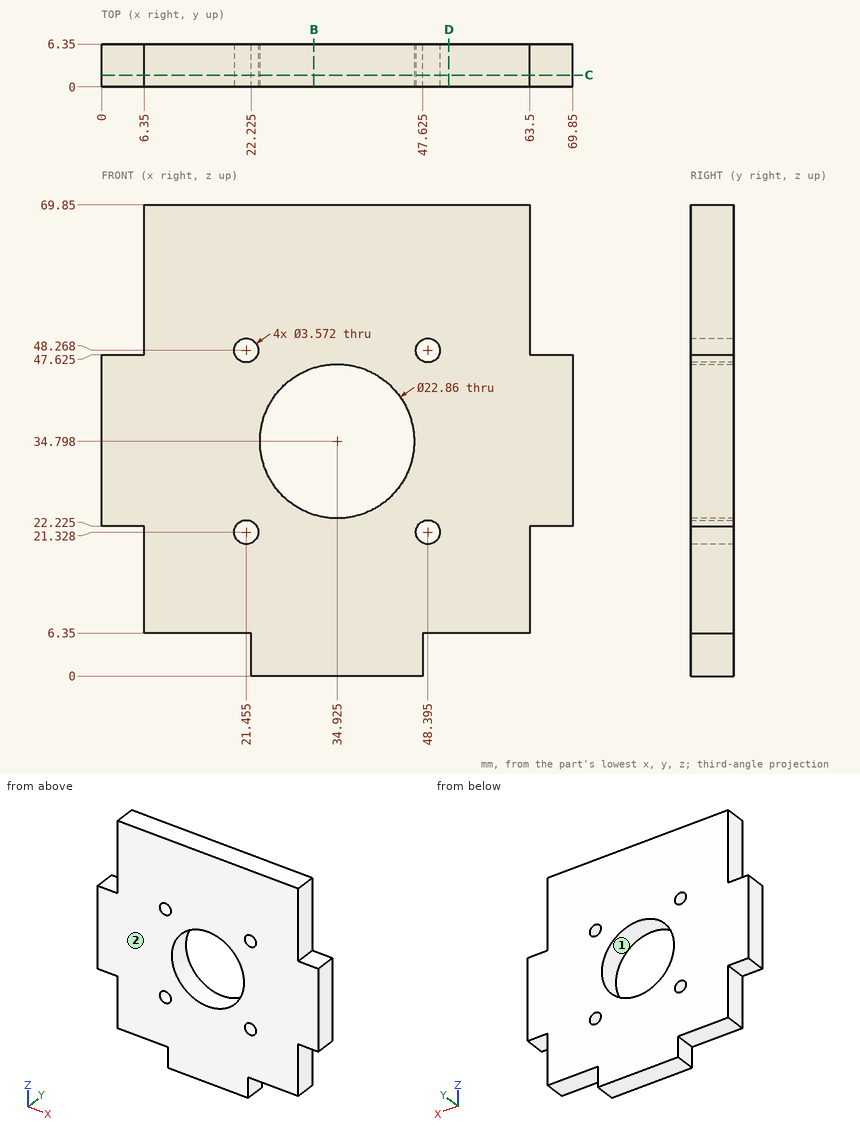
Here's the drawing with two shaded views (mm, measured from the low corner). I have some questions. Coordinates: 2 decimals unless noted, no trailing zeros. Order: outer loops, then holes, each group sorted by start corner. A loop starts at its lowest first (then second) coordinate and runs counter-clockwise, first axis right, second up.
Q1. Suppose I cut it at D-D on x = 51.5. Please give me the cut outline in (y, z), and give its area (3 significant figures).
Q2. Will these pins go through, and if not, where does the flat tip stop? pin 1 (3 mm diameter, centred on x = 21.45, z = 48.27, fed in from +Y); pin 2 (3 mm diameter, centred on x = 67, y = 4, fed in from +Z) (3 decimals); pin 3 (1.9 mm diameter, centred on x = 3.5, y = 4, fed in from -Z) (3 decimals); pin 4 (2 mm diameter, centred on y = 2.5, z = 54.5, fed in from -X).
Q3. Thinking about a two-plate mould opening in X: for the marked faces 1 and 2, which applies, released by +X, released by -X, zero draft, split by the parting line, or undercut?
Q4. Suppose I cut it at C-C on y = 1.75. Give the number of separate pieces and of enclosed holes in the cut face, and give its area (3 significant figures).
Q5. Suppose I cut it at B-B on x = 31.5. Please give me the cut outline in (y, z), and give its area (3 significant figures).
Q6. Please list where these lines run through material, in increasing order: L1, parallel to Z at x = 17, y = 5.25; L2, parallel to Z at x = 36.5, y = 1; L3, parallel to X at y = 4.75, z = 45.
Answer:
1. outline: (0, 6.35) - (6.35, 6.35) - (6.35, 69.85) - (0, 69.85) - close
1. area: 403 mm2
2. pin 1: passes through
2. pin 2: stops at z = 47.625
2. pin 3: stops at z = 22.225
2. pin 4: stops at x = 6.35
3. face 1: undercut
3. face 2: zero draft
4. separate pieces: 1
4. enclosed holes: 5
4. area: 3,660 mm2
5. outline: (0, 0) - (6.35, 0) - (6.35, 23.89) - (0, 23.89) - close; (0, 45.7) - (6.35, 45.7) - (6.35, 69.85) - (0, 69.85) - close
5. area: 305 mm2
6. L1: z = 6.35 to 69.85
6. L2: z = 0 to 23.48, 46.12 to 69.85
6. L3: x = 0 to 29.77, 40.08 to 69.85
